Here's how the part is built. I have some questions about the finished solid (model axes, mm). Round coordinates to 2 decimals unless told otherwise and drop trailing zeros. Loops run counter-clockwise (first coordinate to the right, second up) from the corner with the lowest first, then second, coordinate; pieces in that order, holes last. Notation, with made-up numbers: (1.25, 43.5) - (30.25, 43.5) arc R11 ccw to (30.25, 61.5) - close; hole circle Ø8 at (36, 55). An arc over 180 degrees is marked (long way). Answer as a JSON object with one key per item and string values. Group by question number.
1) I want a section at B-B, the plane z = -12.5. Please give me the cut outline in (x, y) (3 decimals), then the cut area to 3 significant figures.
2) I want a section at C-C, the plane x = 37.5. Please give me the cut outline in (y, z).
3) Will these pins go through, and if not, where does the flat tip stop? P1, Ø1, axis at y = -69, z = -4.5, coming from the -X side; P2, Ø8, axis at x = 17.5, z = -42.5, coming from the +Y side.
4) I want a section at A-A, the plane x = -37.5. Please give me the cut outline in (y, z).
5) If I drill on line 1 along X through (y, z) = (-70, -14) (3 decimals); line 2 along X through (y, z) = (-70.3, -6) (3 decimals); line 3 along Z through (x, y) = (-19, -70.1), over which ranges is the centre line in solid material (lowest first)? Write a range as [from, to].
6) I want a section at D-D, the plane x = -20.5. Please give me the cut outline in (y, z), then the cut area to 3 significant figures.
from build123d import *

# Parameters (mm, degrees)
BOSS_EXTRUDE1_DEPTH = 2.2


with BuildPart() as part:
    # Sketch1 → Boss-Extrude1 (new body)
    with BuildSketch(Plane(origin=(0, -71.98718802, -2.513847999), x_dir=(1, 0, 0), z_dir=(0, -0.9993908270190958, -0.034899496702501066))):
        with BuildLine():
            Line((-53.175, -49.240365792), (53.175, -49.240365792))
            ThreePointArc((53.175, -49.240365792), (54.589213562, -48.654579354), (55.175, -47.240365792))
            Line((55.175, -47.240365792), (55.175, 2.21159528))
            ThreePointArc((55.175, 2.21159528), (54.589213562, 3.625808843), (53.175, 4.21159528))
            Line((53.175, 4.21159528), (-53.175, 4.21159528))
            ThreePointArc((-53.175, 4.21159528), (-54.589213562, 3.625808843), (-55.175, 2.21159528))
            Line((-55.175, 2.21159528), (-55.175, -47.240365792))
            ThreePointArc((-55.175, -47.240365792), (-54.589213562, -48.654579354), (-53.175, -49.240365792))
        make_face()
        with BuildLine():
            Line((-22.025, -32.562401314), (-22.025, -6.262401314))
            ThreePointArc((-22.025, -6.262401314), (-22.903679656, -4.14108097), (-25.025, -3.262401314))
            Line((-25.025, -3.262401314), (-43.325, -3.262401314))
            ThreePointArc((-43.325, -3.262401314), (-45.446320344, -4.14108097), (-46.325, -6.262401314))
            Line((-46.325, -6.262401314), (-46.325, -32.562401314))
            ThreePointArc((-46.325, -32.562401314), (-45.446320344, -34.683721657), (-43.325, -35.562401314))
            Line((-43.325, -35.562401314), (-25.025, -35.562401314))
            ThreePointArc((-25.025, -35.562401314), (-22.903679656, -34.683721657), (-22.025, -32.562401314))
        make_face(mode=Mode.SUBTRACT)
        with BuildLine():
            Line((-8.95, -3.112401314), (8.15, -3.112401314))
            ThreePointArc((8.15, -3.112401314), (10.978427125, -4.283974189), (12.15, -7.112401314))
            Line((12.15, -7.112401314), (12.15, -31.712401314))
            ThreePointArc((12.15, -31.712401314), (10.978427125, -34.540828439), (8.15, -35.712401314))
            Line((8.15, -35.712401314), (-8.95, -35.712401314))
            ThreePointArc((-8.95, -35.712401314), (-11.778427125, -34.540828439), (-12.95, -31.712401314))
            Line((-12.95, -31.712401314), (-12.95, -7.112401314))
            ThreePointArc((-12.95, -7.112401314), (-11.778427125, -4.283974189), (-8.95, -3.112401314))
        make_face(mode=Mode.SUBTRACT)
        with BuildLine():
            Line((25.225, -3.112401314), (42.325, -3.112401314))
            ThreePointArc((42.325, -3.112401314), (45.153427125, -4.283974189), (46.325, -7.112401314))
            Line((46.325, -7.112401314), (46.325, -31.712401314))
            ThreePointArc((46.325, -31.712401314), (45.153427125, -34.540828439), (42.325, -35.712401314))
            Line((42.325, -35.712401314), (25.225, -35.712401314))
            ThreePointArc((25.225, -35.712401314), (22.396572875, -34.540828439), (21.225, -31.712401314))
            Line((21.225, -31.712401314), (21.225, -7.112401314))
            ThreePointArc((21.225, -7.112401314), (22.396572875, -4.283974189), (25.225, -3.112401314))
        make_face(mode=Mode.SUBTRACT)
    extrude(amount=-BOSS_EXTRUDE1_DEPTH)


solid = part.part
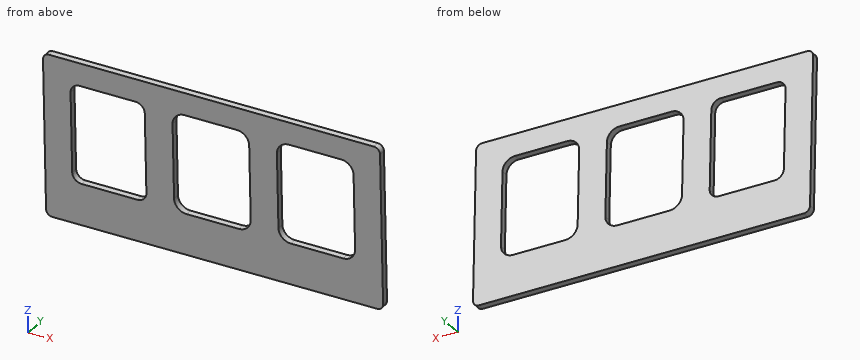
Outcome:
{
 "1": {"outline": "(-55.175, -71.638) - (-46.325, -71.638) - (-46.325, -69.437) - (-55.175, -69.437) - close; (-22.025, -71.638) - (-12.95, -71.638) - (-12.95, -69.437) - (-22.025, -69.437) - close; (12.15, -71.638) - (21.225, -71.638) - (21.225, -69.437) - (12.15, -69.437) - close; (46.325, -71.638) - (55.175, -71.638) - (55.175, -69.437) - (46.325, -69.437) - close", "area": "78.9 mm^2"},
 "2": {"outline": "(-72.13, 1.7) - (-71.88, -5.62) - (-69.68, -5.55) - (-69.94, 1.77) - close; (-70.74, -38.2) - (-70.27, -51.72) - (-68.07, -51.65) - (-68.54, -38.13) - close"},
 "3": {"P1": "through", "P2": "y = -68.25"},
 "4": {"outline": "(-72.13, 1.7) - (-71.87, -5.77) - (-69.67, -5.7) - (-69.94, 1.77) - close; (-70.75, -38.05) - (-70.27, -51.72) - (-68.07, -51.65) - (-68.55, -37.98) - close"},
 "5": {"line 1": "[-55.175, -46.325], [-22.025, -12.95], [12.15, 21.225], [46.325, 55.175]", "line 2": "[-55.175, -44.592], [-23.758, -10.755], [9.955, 23.42], [44.13, 55.175]", "line 3": "[-51.72, 1.77]"},
 "6": {"outline": "(-72.13, 1.7) - (-70.27, -51.72) - (-68.07, -51.65) - (-69.94, 1.77) - close", "area": "118 mm^2"}
}
